```python
from build123d import *

# Parameters (mm, degrees)
SKETCH_1_R      = 11.25
EXTRUDE_2_DEPTH = 3.5


with BuildPart() as part:
    # Эскиз1 → Бобышка-Вытянуть2 (new body)
    with BuildSketch(Plane.XY):
        with BuildLine():
            Line((-15, 16), (15, 16))
            ThreePointArc((15, 16), (15.707106781, 15.707106781), (16, 15))
            Line((16, 15), (16, -15))
            ThreePointArc((16, -15), (15.707106781, -15.707106781), (15, -16))
            Line((15, -16), (-15, -16))
            ThreePointArc((-15, -16), (-15.707106781, -15.707106781), (-16, -15))
            Line((-16, -15), (-16, 15))
            ThreePointArc((-16, 15), (-15.707106781, 15.707106781), (-15, 16))
        make_face()
        Circle(SKETCH_1_R, mode=Mode.SUBTRACT)
        Polygon((-7.272256615, 11.313708499), (-9.292982557, 14.813708499), (-13.334434441, 14.813708499), (-15.355160383, 11.313708499), (-13.334434441, 7.813708499), (-9.292982557, 7.813708499), align=None, mode=Mode.SUBTRACT)
        Polygon((7.272859896, 11.243880856), (9.353756711, 7.779317134), (13.394605314, 7.849144778), (15.354557102, 11.383536142), (13.273660287, 14.848099864), (9.232811684, 14.77827222), align=None, mode=Mode.SUBTRACT)
        Polygon((-7.272256615, -11.313708499), (-9.292982557, -7.813708499), (-13.334434441, -7.813708499), (-15.355160383, -11.313708499), (-13.334434441, -14.813708499), (-9.292982557, -14.813708499), align=None, mode=Mode.SUBTRACT)
        Polygon((15.355160383, -11.313708499), (13.334434441, -7.813708499), (9.292982557, -7.813708499), (7.272256615, -11.313708499), (9.292982557, -14.813708499), (13.334434441, -14.813708499), align=None, mode=Mode.SUBTRACT)
    extrude(amount=EXTRUDE_2_DEPTH)


solid = part.part
```
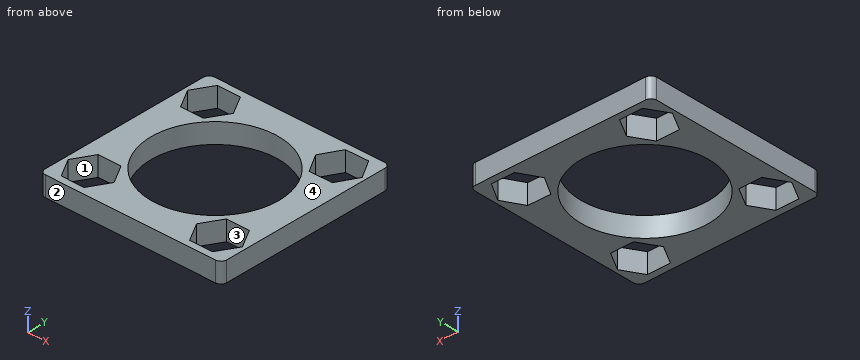
Model file for the job. Use its own axes, mm. Face numbers are marked on the shaded views. A direction names the side the tool comes from. Round coordinates to 2 decimals unless told otherwise and drop trailing zeros. Write each loop counter-clockwise with the first axis right and the second up, starting at its lowest first coordinate (ties: lowest second). Pieces come first, ordered by that corner, then holes. Notation, with made-up numbers: (-25, -6) - (34, -6) arc R33 cw to (34, 27) - close; hole circle Ø2 at (87, 20). An arc over 180 degrees is marked (long way). One line per item, written item: value.
(1) Cut at C-C, the plane x = 10.5. Give the cut face in (y, z), plus the area to 3 significant figures.
Values follow:
outline: (-16, 0) - (-14.81, 0) - (-14.81, 3.5) - (-16, 3.5) - close; (-7.81, 0) - (-4.04, 0) - (-4.04, 3.5) - (-7.81, 3.5) - close; (4.04, 0) - (7.8, 0) - (7.8, 3.5) - (4.04, 3.5) - close; (14.8, 0) - (16, 0) - (16, 3.5) - (14.8, 3.5) - close
area: 34.7 mm²
(2) Cut at A-A, the plane x = 0. Give the cut face in (y, z).
Values follow:
outline: (-16, 0) - (-11.25, 0) - (-11.25, 3.5) - (-16, 3.5) - close; (11.25, 0) - (16, 0) - (16, 3.5) - (11.25, 3.5) - close
(3) Wall check: probe 1 along Y at (x, z) = (13, 2.05); probe 2 along Y at (x, z) = (0, 1.15); probe 3 along X at (y, z) = (14, 2.35). Give the ranges that are in metal, low to high.
Values follow:
probe 1: y = -16 to -14.81, -7.81 to 7.84, 14.84 to 16
probe 2: y = -16 to -11.25, 11.25 to 16
probe 3: x = -16 to -13.8, -8.82 to 8.8, 13.78 to 16
(4) Two-plate mould, pull along X, no slides. Class the marked faces 3 and 4: pulls with the +X half, pulls with the -X half, needs draft (parallel to the pull), parting line crosses it, or undercut.
Values follow:
face 3: undercut
face 4: needs draft
(5) Cut at D-D, the plane z = 0.8. Give the number of separate pieces and of enclosed holes in the cut face, plus the area to 3 significant figures.
Values follow:
separate pieces: 1
enclosed holes: 5
area: 456 mm²
(6) 3-axis set-ups, long thin cutter, end or side, ignore diameter. For the marked faces 1 and 2: which of +Z, -Z, +X, -X, +Y, -Y reach the whole face in a straight line?
Values follow:
face 1: +Z, -Z
face 2: +Z, -Z, +X, -X, -Y
(7) Cut at B-B, the plane y = 9.5. Give the cut face in (x, z), plus the area to 3 significant figures.
Values follow:
outline: (-16, 0) - (-14.31, 0) - (-14.31, 3.5) - (-16, 3.5) - close; (-8.32, 0) - (-6.03, 0) - (-6.03, 3.5) - (-8.32, 3.5) - close; (6.03, 0) - (8.32, 0) - (8.32, 3.5) - (6.03, 3.5) - close; (14.31, 0) - (16, 0) - (16, 3.5) - (14.31, 3.5) - close
area: 27.9 mm²
(8) Drop flat-ended pins along their axis: P1, Ø10, axis at x = -10.5, y = 12, coming from the -Z side; P2, Ø1.5, axis at x = 9, y = 1, coming from the -Z side. Give the stop position or say it passes through.
Values follow:
P1: stops at z = 0
P2: passes through
